Autodesk Fusion 360 part; units mm, degrees
sketch "Front" plane through (0, 0, 0) normal (0, 1, 0) x (1, 0, 0) in component "1006349"
  line L0 (-57.8768, -199.5135) -> (216.2733, -199.5135) construction
  line L1 (-57.6388, 3.5595) -> (225.0785, 3.5595) construction
  line L2 (7.3291, 79.7924) -> (7.3291, -206.2565) construction
  line L3 (213.5386, 80.0304) -> (213.5386, -202.9248) construction
  line L4 (-45.264, -185.7975) -> (221.5088, -185.7975) construction
  line L5 (-43.8142, -9.9025) -> (216.9872, -9.9025) construction
  line L6 (20.1798, 68.3695) -> (20.1798, -205.3046) construction
  line L7 (-33.6031, -100.5805) -> (90.6212, -100.5805) construction
  line L8 (-21.4662, -86.8645) -> (74.9147, -86.8645) construction
  line L9 (51.7406, 52.901) -> (51.7406, -104.1642) construction
  line L10 (64.9486, 43.6199) -> (64.9486, -104.4021) construction
  line L11 (61.3164, 31.245) -> (61.3164, -104.4021) construction
  line L12 (204.2676, 28.1453) -> (204.2676, -293.7347) construction
  line L13 (301.4692, -174.3675) -> (-2.19, -174.3675) construction
  line L14 (289.3324, -128.6475) -> (193.4275, -128.6475) construction
  line L15 (188.2402, -212.6819) -> (188.2402, 15.0626) construction
  line L16 (141.5042, -224.3428) -> (141.5042, 9.827) construction
  line L17 (79.2234, -236.9556) -> (79.2234, 11.9688) construction
  line L18 (32.4366, -262.9987) -> (32.4366, -64.0809) construction
  line L19 (55.2966, -250.3288) -> (55.2966, 19.8573) construction
  line L20 (276.3559, -113.1535) -> (-0.7101, -113.1535) construction
  line L21 (251.1435, -82.9275) -> (47.1227, -82.9275) construction
  line L22 (224.557, -21.7135) -> (42.5012, -21.7135) construction
  line L23 (328.6587, -0.2505) -> (74.127, -0.2505) construction
  line L24 (326.747, -5.7115) -> (-6.8013, -5.7115) construction
  line L25 (238.6648, -67.4335) -> (193.169, -67.4335) construction
  line L26 (209.7286, -275.7982) -> (209.7286, -12.1057) construction
  line L27 (313.957, -195.7035) -> (25.5151, -195.7035) construction
  line L28 (325.8246, -190.0139) -> (-1.5489, -190.0139) construction
  line L29 (263.2084, -90.6745) -> (24.7432, -90.6745) construction
  line L30 (10.999, -276.0365) -> (10.999, -104.4195) construction
  line L31 (16.7648, -288.1351) -> (16.7648, -78.75) construction
  line L32 (7.3291, -199.5135) -> (213.5386, -199.5135)
  line L33 (213.5386, 3.5595) -> (51.7406, 3.5595)
  line L34 (51.7406, -86.8645) -> (51.7406, 3.5595)
  line L35 (51.7406, -86.8645) -> (7.3291, -86.8645)
  line L36 (7.3291, -86.8645) -> (7.3291, -199.5135)
  line L37 (213.5386, -199.5135) -> (213.5386, 3.5595)
  line L38 (20.1798, -104.5315) -> (20.1798, -100.5805)
  line L39 (200.0766, -193.5194) -> (200.0766, 68.0398) construction
  line L40 (-6.7988, -96.9737) -> (70.6703, -96.9737) construction
  line L41 (20.1798, -185.7975) -> (200.0766, -185.7975)
  line L42 (200.0766, -185.7975) -> (200.0766, -5.7115)
  line L43 (64.9486, -5.7115) -> (64.9486, -100.5805)
  line L44 (64.9486, -100.5805) -> (20.1798, -100.5805)
  line L45 (20.1798, -100.5805) -> (20.1798, -185.7975)
  line L46 (200.0766, -9.9025) -> (64.9486, -9.9025)
  point P0 (10.999, -174.3675)
  point P1 (32.4366, -195.7035)
  point P2 (79.2234, -195.7035)
  point P3 (141.5042, -195.7035)
  point P4 (188.2402, -195.7035)
  point P5 (209.7286, -174.3675)
  point P6 (209.7286, -128.6475)
  point P7 (209.7286, -67.4335)
  point P8 (209.7286, -21.7135)
  point P9 (188.2402, -0.2505)
  point P10 (141.5042, -0.2505)
  point P11 (79.2234, -0.2505)
  point P12 (55.2966, -21.7135)
  point P13 (55.2966, -82.9275)
  point P14 (32.4366, -90.6745)
  point P15 (10.999, -113.1535)
  dimension "d1" = 203.073
  dimension "d2" = 174.117
  dimension "d3" = 128.397
  dimension "d4" = 90.424
  dimension "d5" = 82.677
  dimension "d6" = 67.183
  dimension "d7" = 21.463
  dimension "d8" = 195.453
  dimension "d9" = 90.424
  dimension "d10" = 13.462
  dimension "d14" = 198.7296
  dimension "d15" = 177.292
  dimension "d16" = 154.432
  dimension "d17" = 130.5052
  dimension "d18" = 68.2244
  dimension "d19" = 21.4884
  dimension "d20" = 161.798
  dimension "d22" = 142.9512
  dimension "d26" = 175.895
  dimension "d27" = 112.903
  dimension "d28" = 184.3024
  dimension "d31" = 5.461
  dimension "d32" = 13.716
  dimension "d33" = 187.5028
  dimension "d46" = 9.652
  dimension "d48" = 13.462
  dimension "d49" = 135.128
  dimension "d50" = 91.2622
  dimension "d51" = 5.461
extrude "Extrude2" add sketch "Front" along normal blind 3.175 in component "1006349"
chamfer "Chamfer3" distance 3.556 angle 45 4 edges at (213.5386, 1.5875, -3.5595) (64.9486, 1.5875, 100.5805) (7.3291, 1.5875, 199.5135) (213.5386, 1.5875, 199.5135) in component "1006349"
chamfer "Chamfer4" distance 12.7 angle 45 2 edges at (7.3291, 1.5875, 86.8645) (51.7406, 1.5875, -3.5595) in component "1006349"
fillet "Fillet2" radius 5.5372 6 edges at (20.1798, 1.5875, 185.7975) (20.1798, 1.5875, 100.5805) (64.9486, 1.5875, 9.9025) (200.0766, 1.5875, 9.9025) (200.0766, 1.5875, 185.7975) (51.7406, 1.5875, 86.8645) in component "1006349"
hole "Hole2" at (32.4366, 0, 195.7035) at (79.2234, 0, 195.7035) at (141.5042, 0, 195.7035) at (188.2402, 0, 195.7035) at (10.999, 0, 174.3675) at (10.999, 0, 113.1535) at (32.4366, 0, 90.6745) at (209.7286, 0, 174.3675) at (209.7286, 0, 128.6475) at (209.7286, 0, 67.4335) at (209.7286, 0, 21.7135) at (188.2402, 0, 0.2505) at (141.5042, 0, 0.2505) at (79.2234, 0, 0.2505) at (55.2966, 0, 21.7135) at (55.2966, 0, 82.9275) direction (0, 1, 0) diameter 4.0894 end through all in component "1006349"
component "1006349" placed x (1, 0, 0) y (0, 1, 0) z (0, 0, 1) at (0, 0, 0)
Could you check a few things on this model? Use its own coordinates, in mm. A direction names the side the tool comes from. Give positions to 0.01 mm unless a question says otherwise; leave off trailing zeros. Write each loop counter-clockwise with the first axis right and the second up, starting at its lowest first coordinate (ties: lowest second). Pieces come first, ordered by that corner, then holes. Notation, with made-up numbers: (11, 77.5) - (15, 77.5) arc R7 cw to (15, 84.5) - close; hole circle Ø7 at (57, 22). An arc over 180 degrees is marked (long way). Use CSV: the item, a comma, the result in double quotes. Start each with the question number.
Item 1: I'm going to push flat-ended pins straight in: pin 1 (3.5 mm diameter, centred on x = 79.22, z = 195.7, fed in from -Y); pin 2 (1.6 mm diameter, centred on x = 27.5, y = 2, fed in from -Z). Where does each tip first touch, or does it pass through?
Item 2: If we mould it in two halves opening along X, with no side actions, what happens to faces 1 (the face through (66.614, 1.61, 11.481)), 2 (the face through (63, 0, 97)), 3 (the face through (13.768, 1.565, 93.126))? For each: pulls with the +X half, pulls with the -X half, needs draft (parallel to the pull), parting line crosses it, or undercut.
Item 3: For faces 4 (the face through (198.41, 1.61, 184.22)), 5 (the face through (50.076, 1.61, 85.286)), which set-ups out of +Z, -Z, +X, -X, +Y, -Y let a thin tool reach every point of the face, with its end or its side?
Item 4: I want a section at C-C, the plane y = 1.85. Give the number of separate pieces and of enclosed holes in the cut face, then the cut area to 3 significant figures.
Item 5: I want a section at B-B, the plane z = 155. Please give me the cut outline in (x, y) (3 decimals).
Item 6: I want a section at A-A, the plane x = 113.5. Please give me the cut outline in (y, z) (1 decimal), then the cut area to 3 significant figures.
Item 7: If I drill on line 1 along Z through (x, y) = (156.5, 0.95); line 2 along Z through (x, y) = (79, 0.95); line 3 along X through (y, z) = (0.25, 25.5), over which ranges is the centre line in solid material (lowest first)?
Findings:
1,pin 1,"passes through"
1,pin 2,"stops at z = 86.86"
2,face 1,"undercut"
2,face 2,"needs draft"
2,face 3,"pulls with the -X half"
3,face 4,"+Y, -Y"
3,face 5,"-Z, -X, +Y, -Y"
4,separate pieces,"1"
4,enclosed holes,"17"
4,area,"9,920 mm2"
5,outline,"(7.329, 0) - (20.18, 0) - (20.18, 3.175) - (7.329, 3.175) - close; (200.077, 0) - (213.539, 0) - (213.539, 3.175) - (200.077, 3.175) - close"
6,outline,"(0, -3.6) - (3.2, -3.6) - (3.2, 9.9) - (0, 9.9) - close; (0, 185.8) - (3.2, 185.8) - (3.2, 199.5) - (0, 199.5) - close"
6,area,"86.3 mm2"
7,line 1,"z = -3.56 to 9.9, 185.8 to 199.51"
7,line 2,"z = -3.56 to -1.78, 2.28 to 9.9, 185.8 to 193.67, 197.74 to 199.51"
7,line 3,"x = 51.74 to 64.95, 200.08 to 213.54"
